Could you check a few things on this model? Use its own coordinates, in mm. Coordinates: 2 decimals unless noted, no trailing zeros. Write each loop counter-clockwise with the first axis right and the second up, starting at its lowest first coordinate (ties: lowest second). Pieces come first, ordered by that corner, then holes.
```python
from build123d import *

# Parameters (mm, degrees)
SKIZZE1_W                       = 285
SKIZZE1_H                       = 325
AUFSATZ_LINEAR_AUSTRAGEN1_DEPTH = 5
SKIZZE2_W                       = 5
SKIZZE2_H                       = 100
SCHNITT_LINEAR_AUSTRAGEN1_DEPTH = 433.290411645


with BuildPart() as part:
    # Skizze1 → Aufsatz-Linear austragen1 (new body)
    with BuildSketch(Plane(origin=(0, 0, 0), x_dir=(1, 0, 0), z_dir=(0, 1, 0))):
        with Locations((142.5, 162.5)):
            Rectangle(SKIZZE1_W, SKIZZE1_H)
    extrude(amount=AUFSATZ_LINEAR_AUSTRAGEN1_DEPTH)

    # Skizze2 → Schnitt-Linear austragen1 (cut, through all)
    with BuildSketch(Plane(origin=(0, 5, 0), x_dir=(1, 0, 0), z_dir=(0, 1, 0))):
        Polygon((142.5, 325), (92.5, 325), (92.5, 320), (192.5, 320), (192.5, 325), align=None)
        with Locations((2.5, 162.5)):
            Rectangle(SKIZZE2_W, SKIZZE2_H)
        with Locations((282.5, 162.5)):
            Rectangle(SKIZZE2_W, SKIZZE2_H)
        Polygon((142.5, 0), (192.5, 0), (192.5, 5), (92.5, 5), (92.5, 0), align=None)
    extrude(amount=-SCHNITT_LINEAR_AUSTRAGEN1_DEPTH, mode=Mode.SUBTRACT)


solid = part.part
```
1. I want a section at B-B on x = 119.5. Please give me the cut outline in (y, z), plus the area to 4 significant figures.
Verdict:
outline: (0, -320) - (5, -320) - (5, -5) - (0, -5) - close
area: 1,575 mm2
2. For pin 1 (1.5 mm diameter, centred on y = 2, z = -178.5, fed in from -X); pin 2 (1.5 mm diameter, centred on x = 119.5, y = 3, fed in from -Z), each with a flat end and sliding along its axis, tell me the tip position at first contact or that it passes through.
Verdict:
pin 1: stops at x = 5
pin 2: stops at z = -320
3. I want a section at C-C on z = -146. Please give me the cut outline in (x, y).
Verdict:
outline: (5, 0) - (280, 0) - (280, 5) - (5, 5) - close
4. Please list where these lines run through material, in increasing order: line 1 along Z through (x, y) = (118, 1.4); line 2 along X through (y, z) = (2.2, -207.5).
Verdict:
line 1: z = -320 to -5
line 2: x = 5 to 280
5. I want a section at A-A on y = 2. Please give me the cut outline in (x, z), plus the area to 3 significant figures.
Verdict:
outline: (0, -325) - (92.5, -325) - (92.5, -320) - (192.5, -320) - (192.5, -325) - (285, -325) - (285, -212.5) - (280, -212.5) - (280, -112.5) - (285, -112.5) - (285, 0) - (192.5, 0) - (192.5, -5) - (92.5, -5) - (92.5, 0) - (0, 0) - (0, -112.5) - (5, -112.5) - (5, -212.5) - (0, -212.5) - close
area: 90,600 mm2
